```python
from build123d import *

# Parameters (mm, degrees)
F0_W     = 74.4
F0_H     = 39.6
F0_R     = 1
F0_R_2   = 4.1
F1_DEPTH = 1.5
F2_W     = 25
F2_H     = 1.5
F3_DEPTH = 40
F4_R     = 1
F4_R_2   = 4.1
F5_DEPTH = 1.5
F6_R     = 5


with BuildPart() as f1:
    # F0 (on Top) → F1 (new body)
    with BuildSketch(Plane.XY):
        Rectangle(F0_W, F0_H)
        with Locations((-32.2, -16.8)):
            Circle(F0_R, mode=Mode.SUBTRACT)
        with Locations((-25, -10.6)):
            Circle(F0_R_2, mode=Mode.SUBTRACT)
        with Locations((-17.8, -16.8)):
            Circle(F0_R, mode=Mode.SUBTRACT)
        with Locations((17.8, -16.8)):
            Circle(F0_R, mode=Mode.SUBTRACT)
        with Locations((32.2, -16.8)):
            Circle(F0_R, mode=Mode.SUBTRACT)
        with Locations((25, -10.6)):
            Circle(F0_R_2, mode=Mode.SUBTRACT)
        with BuildLine():
            ThreePointArc((-34.8, 11.6), (-34.507107, 12.307107), (-33.8, 12.6))
            Line((-33.8, 12.6), (-30.123475, 12.6))
            ThreePointArc((-30.123475, 12.6), (-25, 15.1), (-19.876525, 12.6))
            Line((-19.876525, 12.6), (-16.2, 12.6))
            ThreePointArc((-16.2, 12.6), (-15.492893, 12.307107), (-15.2, 11.6))
            Line((-15.2, 11.6), (-15.2, 1.9))
            ThreePointArc((-15.2, 1.9), (-16.664466, -1.635534), (-20.2, -3.1))
            Line((-20.2, -3.1), (-29.8, -3.1))
            ThreePointArc((-29.8, -3.1), (-33.335534, -1.635534), (-34.8, 1.9))
            Line((-34.8, 1.9), (-34.8, 11.6))
        make_face(mode=Mode.SUBTRACT)
        with Locations((-32.2, 14.8)):
            Circle(F0_R, mode=Mode.SUBTRACT)
        with Locations((-17.8, 14.8)):
            Circle(F0_R, mode=Mode.SUBTRACT)
        with BuildLine():
            Line((15.2, 1.9), (15.2, 11.6))
            ThreePointArc((15.2, 11.6), (15.492893, 12.307107), (16.2, 12.6))
            Line((16.2, 12.6), (19.876525, 12.6))
            ThreePointArc((19.876525, 12.6), (25, 15.1), (30.123475, 12.6))
            Line((30.123475, 12.6), (33.8, 12.6))
            ThreePointArc((33.8, 12.6), (34.507107, 12.307107), (34.8, 11.6))
            Line((34.8, 11.6), (34.8, 1.9))
            ThreePointArc((34.8, 1.9), (33.335534, -1.635534), (29.8, -3.1))
            Line((29.8, -3.1), (20.2, -3.1))
            ThreePointArc((20.2, -3.1), (16.664466, -1.635534), (15.2, 1.9))
        make_face(mode=Mode.SUBTRACT)
        with Locations((17.8, 14.8)):
            Circle(F0_R, mode=Mode.SUBTRACT)
        with Locations((32.2, 14.8)):
            Circle(F0_R, mode=Mode.SUBTRACT)
    extrude(amount=F1_DEPTH)

    # F2 (on Top) → F3 (join)
    with BuildSketch(Plane.XY):
        with Locations((0, 20.55)):
            Rectangle(F2_W, F2_H)
    extrude(amount=F3_DEPTH)

    # F4 (on face) → F5 (cut, through all)
    with BuildSketch(Plane(origin=(0, 21.3, 0), x_dir=(-1, 0, 0), z_dir=(0, 1, 0))):
        with Locations((7.2, 37)):
            Circle(F4_R)
        with Locations((7.2, 5.4)):
            Circle(F4_R)
        with Locations((0, 11.6)):
            Circle(F4_R_2)
        with BuildLine():
            ThreePointArc((9.8, 33.9), (9.507107, 34.607107), (8.8, 34.9))
            Line((8.8, 34.9), (5.499091, 34.9))
            ThreePointArc((5.499091, 34.9), (5.099091, 34.983485), (4.765879, 35.22))
            ThreePointArc((4.765879, 35.22), (0, 37.3), (-4.765879, 35.22))
            ThreePointArc((-4.765879, 35.22), (-5.099091, 34.983485), (-5.499091, 34.9))
            Line((-5.499091, 34.9), (-8.8, 34.9))
            ThreePointArc((-8.8, 34.9), (-9.507107, 34.607107), (-9.8, 33.9))
            Line((-9.8, 33.9), (-9.8, 24.2))
            ThreePointArc((-9.8, 24.2), (-8.335534, 20.664466), (-4.8, 19.2))
            Line((-4.8, 19.2), (4.8, 19.2))
            ThreePointArc((4.8, 19.2), (8.335534, 20.664466), (9.8, 24.2))
            Line((9.8, 24.2), (9.8, 33.9))
        make_face()
        with Locations((-7.2, 37)):
            Circle(F4_R)
        with Locations((-7.2, 5.4)):
            Circle(F4_R)
    extrude(amount=-F5_DEPTH, mode=Mode.SUBTRACT)

    # F6
    f6_edges = [f1.edges().sort_by_distance(p)[0] for p in [
        (-37.2, 19.8, 0.75),
        (-37.2, -19.8, 0.75),
        (37.2, 19.8, 0.75),
        (37.2, -19.8, 0.75),
        (-12.5, 20.55, 40),
        (12.5, 20.55, 40),
    ]]
    fillet(f6_edges, radius=F6_R)


solid = f1.part
```
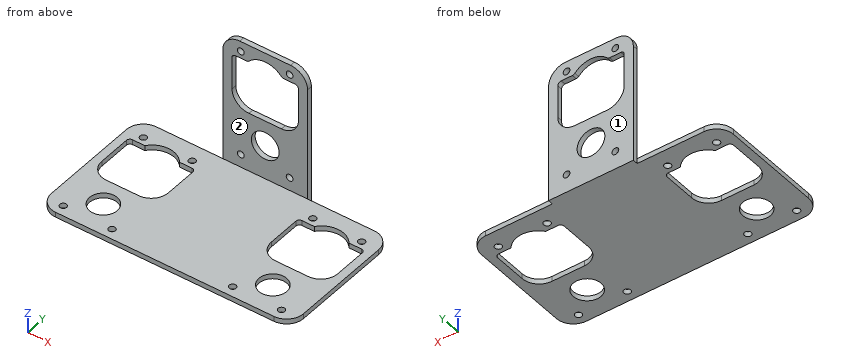
CAD build for the part. Positions are in the model's coordinates, mm. Face numbers are marked on the shaded views. A direction names the side the tool comes from. Round coordinates to 2 decimals unless told otherwise and drop trailing zeros. Order: outer loops, then holes, each group sorted by start corner. A loop starts at its lowest first (then second) coordinate and runs counter-clockwise, first axis right, second up.
Item 1: Pin check, flat tips, straight feed: pin 1 (1.6 mm diameter, centred on y = 21, z = 30, fed in from -X); pin 2 (7.5 mm diameter, centred on x = -1.5, z = 22, fed in from -Y); pin 3 (12 mm diameter, centred on y = 15, z = 12, fed in from +X). Stop position of each tip, or through.
Item 2: Probe line 1 along Z through (x, y) = (7.2, 20.3); line 2 along Y through (x, z) = (-17.8, 1.05); line 3 along Z through (x, y) = (-22, -13.5). List the from-to ranges inside material, lowest first.
Item 3: Saw through at C-C on z = 5.4. Write the cut outline in (x, y), then the cut area to 3 significant figures.
Item 4: Tool access for the marked faces 1 and 2: list every direction of +Z, -Z, +X, -X, +Y, -Y with a clear straight run to the whole face (end or side of a thin tool).
Item 5: Saw through at D-D on z = 10.5. Write the cut outline in (x, y), then the cut area to 3 significant figures.
Item 6: Saw through at A-A on y = -10.6. Write the cut outline in (x, z), then the cut area to 3 significant figures.
Item 7: Saw through at B-B on x = 0. Write the cut outline in (y, z), then the cut area to 4 significant figures.
Reported:
1. pin 1: stops at x = -12.5
1. pin 2: stops at y = 19.8
1. pin 3: stops at x = 12.5
2. line 1: z = 0 to 4.4, 6.4 to 19.81, 34.9 to 36, 38 to 40
2. line 2: y = -19.8 to -17.8, -15.8 to -2.49, 12.6 to 13.8, 15.8 to 19.8
2. line 3: z = 0 to 1.5
3. outline: (-12.5, 19.8) - (-8.2, 19.8) - (-8.2, 21.3) - (-12.5, 21.3) - close; (-6.2, 19.8) - (6.2, 19.8) - (6.2, 21.3) - (-6.2, 21.3) - close; (8.2, 19.8) - (12.5, 19.8) - (12.5, 21.3) - (8.2, 21.3) - close
3. area: 31.5 mm2
4. face 1: +Z, -Z, +X, -X, +Y
4. face 2: +Z, +X, -X, -Y
5. outline: (-12.5, 19.8) - (-3.95, 19.8) - (-3.95, 21.3) - (-12.5, 21.3) - close; (3.95, 19.8) - (12.5, 19.8) - (12.5, 21.3) - (3.95, 21.3) - close
5. area: 25.7 mm2
6. outline: (-37.2, 0) - (-29.1, 0) - (-29.1, 1.5) - (-37.2, 1.5) - close; (-20.9, 0) - (20.9, 0) - (20.9, 1.5) - (-20.9, 1.5) - close; (29.1, 0) - (37.2, 0) - (37.2, 1.5) - (29.1, 1.5) - close
6. area: 87.0 mm2
7. outline: (-19.8, 0) - (21.3, 0) - (21.3, 7.5) - (19.8, 7.5) - (19.8, 1.5) - (-19.8, 1.5) - close; (19.8, 15.7) - (21.3, 15.7) - (21.3, 19.2) - (19.8, 19.2) - close; (19.8, 37.3) - (21.3, 37.3) - (21.3, 40) - (19.8, 40) - close
7. area: 79.95 mm2
